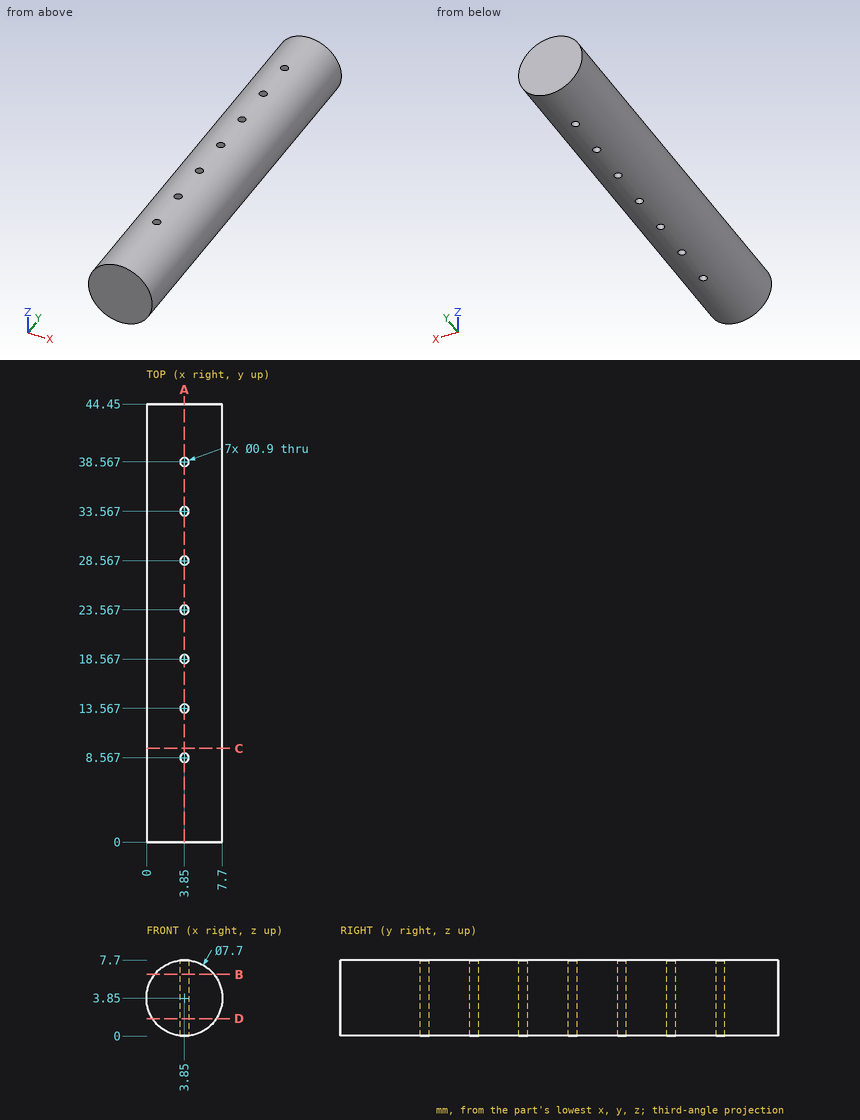
Could you check a few things on this drawing? It's one solid part, dimensions in mm from its lowest x, y, z. Coordinates: 2 decimals unless noted, no trailing zeros. Write each loop counter-clockwise with the first axis right and the second up, starting at its lowest first coordinate (ties: lowest second). Pieces come first, ordered by that corner, then holes. Notation, with made-up numbers: (62.25, 4) - (101.25, 4) arc R23 ccw to (101.25, 33) - close; hole circle Ø8 at (61, 27). An arc over 180 degrees is marked (long way). Use one line per item in the form item = value.
1) Suppose I cut it at C-C, the plane y = 9.5. Write out the boundary of the cut face in (x, z).
Solved:
outline = circle Ø7.7 at (3.85, 3.85)
2) I need wall thicknesses on line 1 (X direction, y = 40.5, z = 4); line 2 (Z direction, x = 6.25, y = 29.5); line 3 (Z direction, x = 3.25, y = 24). Which ranges of each line are inside material? Lowest first, please.
Solved:
line_1 = 0 to 7.7
line_2 = 0.84 to 6.86
line_3 = 0.05 to 7.65
3) Suppose I cut it at B-B, the plane z = 6.25. Write out the boundary of the cut face in (x, y).
Solved:
outline = (0.84, 0) - (6.86, 0) - (6.86, 44.45) - (0.84, 44.45) - close; hole circle Ø0.9 at (3.85, 8.57); hole circle Ø0.9 at (3.85, 13.57); hole circle Ø0.9 at (3.85, 18.57); hole circle Ø0.9 at (3.85, 23.57); hole circle Ø0.9 at (3.85, 28.57); hole circle Ø0.9 at (3.85, 33.57); hole circle Ø0.9 at (3.85, 38.57)
4) Suppose I cut it at A-A, the plane x = 3.85. Give the number of separate pieces and of enclosed holes in the cut face, plus the area to 3 significant figures.
Solved:
separate_pieces = 8
enclosed_holes = 0
area = 294 mm2
5) Suppose I cut it at D-D, the plane z = 1.75. Write out the boundary of the cut face in (x, y).
Solved:
outline = (0.62, 0) - (7.08, 0) - (7.08, 44.45) - (0.62, 44.45) - close; hole circle Ø0.9 at (3.85, 8.57); hole circle Ø0.9 at (3.85, 13.57); hole circle Ø0.9 at (3.85, 18.57); hole circle Ø0.9 at (3.85, 23.57); hole circle Ø0.9 at (3.85, 28.57); hole circle Ø0.9 at (3.85, 33.57); hole circle Ø0.9 at (3.85, 38.57)
6) I'm going to push flat-ended pins straight in: P1, Ø3, axis at y = 38.5, z = 6.5, coming from the +X side; P2, Ø1.5, axis at y = 30, z = 6, coming from the +X side; P3, Ø1.5, axis at x = 6, y = 18, coming from the +Z side. Where does each tip first touch, or does it pass through?
Solved:
P1 = 7.52
P2 = 7.44
P3 = 7.44
